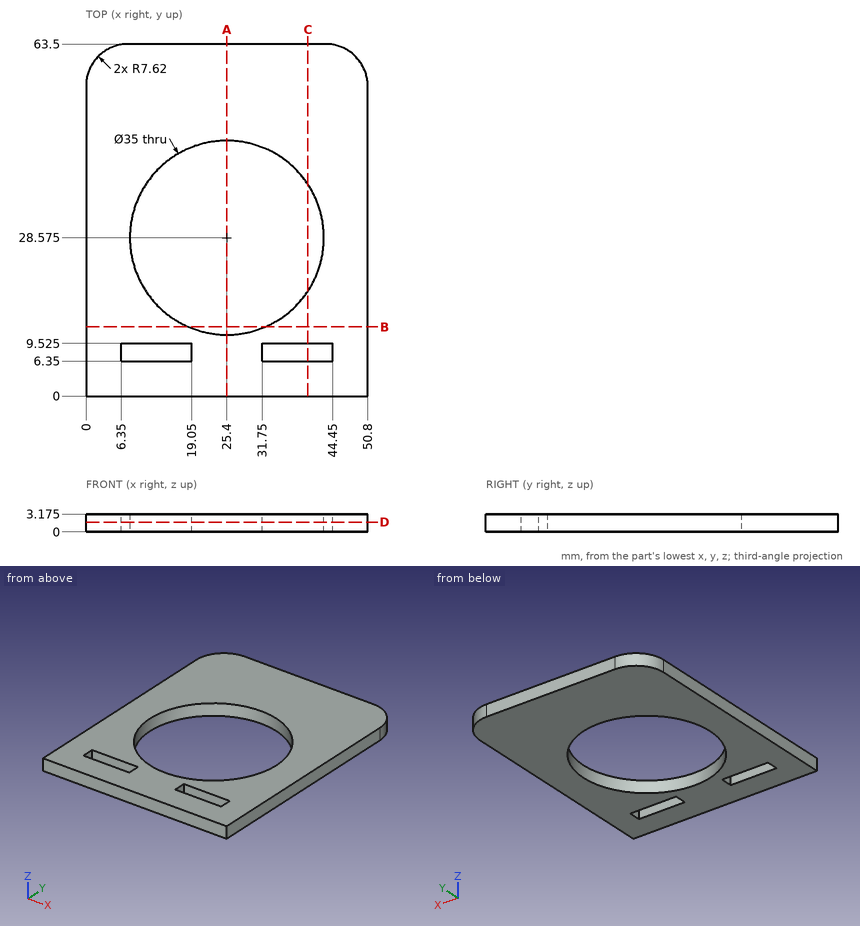
Job drawing, mm, ordinate dimensions from the low corner. One solid piece. Round coordinates to 2 decimals unless told otherwise and drop trailing zeros. Order: outer loops, then holes, each group sorted by start corner. A loop starts at its lowest first (then second) coordinate and runs counter-clockwise, first axis right, second up. Notation, with made-up numbers: (50.25, 26) - (100.25, 26) arc R3 cw to (100.25, 30) - close; hole circle Ø5 at (-11.75, 46). An arc over 180 degrees is marked (long way). Use CSV: the item, a comma, the result in double quotes. Start each with the question number.
1) Saw through at A-A (x = 25.4). List the corners of the cut face in (y, z) (3 decimals).
2) Saw through at D-D (z = 1.75). List the corners of the cut face in (x, y) (3 decimals), and give its area (3 significant figures).
3) Saw through at B-B (y = 12.5). List the corners of the cut face in (x, z) (3 decimals).
4) Wall check: L1, parallel to Y at x = 25.4, z = 1.15 (3 decimals); L2, parallel to Y at x = 40, z = 3 (3 decimals); L3, parallel to X at y = 7, z = 0.2. Give the ranges that are in metal, low to high. Write a range as [from, to].
5) Saw through at C-C (x = 40). List the corners of the cut face in (y, z) (3 decimals).
6) Pin check, flat tip, straight feed: pin 1 Ø8 at (x, y) = (26.5, 44) entering from -Z. Stop position of the tip, or through.
Values follow:
1,outline,"(0, 0) - (11.075, 0) - (11.075, 3.175) - (0, 3.175) - close; (46.075, 0) - (63.5, 0) - (63.5, 3.175) - (46.075, 3.175) - close"
2,outline,"(0, 0) - (50.8, 0) - (50.8, 55.88) arc R7.62 ccw to (43.18, 63.5) - (7.62, 63.5) arc R7.62 ccw to (0, 55.88) - close; hole (6.35, 6.35) - (19.05, 6.35) - (19.05, 9.525) - (6.35, 9.525) - close; hole circle Ø35 at (25.4, 28.575); hole (31.75, 6.35) - (44.45, 6.35) - (44.45, 9.525) - (31.75, 9.525) - close"
2,area,"2,160 mm2"
3,outline,"(0, 0) - (18.483, 0) - (18.483, 3.175) - (0, 3.175) - close; (32.317, 0) - (50.8, 0) - (50.8, 3.175) - (32.317, 3.175) - close"
4,L1,"y = [0, 11.075], [46.075, 63.5]"
4,L2,"y = [0, 6.35], [9.525, 18.927], [38.223, 63.5]"
4,L3,"x = [0, 6.35], [19.05, 31.75], [44.45, 50.8]"
5,outline,"(0, 0) - (6.35, 0) - (6.35, 3.175) - (0, 3.175) - close; (9.525, 0) - (18.927, 0) - (18.927, 3.175) - (9.525, 3.175) - close; (38.223, 0) - (63.5, 0) - (63.5, 3.175) - (38.223, 3.175) - close"
6,pin 1,"stops at z = 0"
